from build123d import *

# Parameters (mm, degrees)
SKETCH1_R           = 1.720095417
SKETCH1_R_2         = 1.632335783
BOSS_EXTRUDE1_DEPTH = 2.54


with BuildPart() as part:
    # Sketch1 → Boss-Extrude1 (new body)
    with BuildSketch(Plane.XY):
        with BuildLine():
            Line((0.359622665, 84.647626996), (0.359622665, 112.547896558))
            ThreePointArc((0.359622665, 112.547896558), (1.569792033, 115.17822767), (4.285435965, 116.18243367))
            Line((4.285435965, 116.18243367), (699.960441306, 116.18243367))
            Line((699.960441306, 116.18243367), (699.960441306, 131.904163347))
            ThreePointArc((699.960441306, 131.904163347), (701.183091811, 134.700225562), (704.024750828, 135.812795653))
            Line((704.024750828, 135.812795653), (857.125984653, 135.812795653))
            Line((857.125984653, 135.812795653), (857.125984653, 124.543323228))
            Line((857.125984653, 124.543323228), (714.00720644, 124.543323228))
            Line((714.00720644, 124.543323228), (714.00720644, 104.995667719))
            Line((714.00720644, 104.995667719), (12.71320644, 104.995667719))
            Line((12.71320644, 104.995667719), (12.71320644, 91.663924817))
            Line((12.71320644, 91.663924817), (714.00720644, 91.663924817))
            Line((714.00720644, 91.663924817), (714.00720644, 72.51225313))
            Line((714.00720644, 72.51225313), (935.984655082, 72.51225313))
            Line((935.984655082, 72.51225313), (935.984655082, 124.543323228))
            Line((935.984655082, 124.543323228), (933.071984653, 124.543323228))
            Line((933.071984653, 124.543323228), (933.071984653, 135.812795653))
            Line((933.071984653, 135.812795653), (946.192785632, 135.812795653))
            ThreePointArc((946.192785632, 135.812795653), (948.657072186, 134.878542119), (949.738968911, 132.475411377))
            Line((949.738968911, 132.475411377), (949.738968911, 64.012598058))
            ThreePointArc((949.738968911, 64.012598058), (948.74540471, 61.39621374), (946.192785632, 60.24870663))
            Line((946.192785632, 60.24870663), (704.024750828, 60.24870663))
            ThreePointArc((704.024750828, 60.24870663), (701.213068629, 61.288906282), (699.960441306, 64.012598058))
            Line((699.960441306, 64.012598058), (699.960441306, 81.011908201))
            Line((699.960441306, 81.011908201), (4.285435965, 81.011908201))
            ThreePointArc((4.285435965, 81.011908201), (1.569547298, 82.016705042), (0.359622665, 84.647626996))
        make_face()
        with Locations((94.1622142, 88.091107164)):
            Circle(SKETCH1_R, mode=Mode.SUBTRACT)
        with Locations((94.1622142, 108.484732819)):
            Circle(SKETCH1_R, mode=Mode.SUBTRACT)
        with Locations((221.392126764, 108.484732819)):
            Circle(SKETCH1_R, mode=Mode.SUBTRACT)
        with Locations((221.392126764, 88.091107164)):
            Circle(SKETCH1_R, mode=Mode.SUBTRACT)
        with Locations((348.078760153, 108.484732819)):
            Circle(SKETCH1_R, mode=Mode.SUBTRACT)
        with Locations((348.078760153, 88.091107164)):
            Circle(SKETCH1_R_2, mode=Mode.SUBTRACT)
        with Locations((475.146430575, 108.484732819)):
            Circle(SKETCH1_R, mode=Mode.SUBTRACT)
        with Locations((475.146430575, 88.091107164)):
            Circle(SKETCH1_R, mode=Mode.SUBTRACT)
        with Locations((602.130384222, 88.091107164)):
            Circle(SKETCH1_R, mode=Mode.SUBTRACT)
        with Locations((602.130384222, 108.484732819)):
            Circle(SKETCH1_R, mode=Mode.SUBTRACT)
        with Locations((705.892847696, 116.18243367)):
            Circle(SKETCH1_R, mode=Mode.SUBTRACT)
        with Locations((705.892847696, 81.011908201)):
            Circle(SKETCH1_R, mode=Mode.SUBTRACT)
        with Locations((760.070975046, 130.611938178)):
            Circle(SKETCH1_R, mode=Mode.SUBTRACT)
        with Locations((760.070975046, 66.505299661)):
            Circle(SKETCH1_R, mode=Mode.SUBTRACT)
        with Locations((848.138968911, 130.611938178)):
            Circle(SKETCH1_R, mode=Mode.SUBTRACT)
        with Locations((848.138968911, 66.505299661)):
            Circle(SKETCH1_R, mode=Mode.SUBTRACT)
        with Locations((943.890172073, 116.18243367)):
            Circle(SKETCH1_R, mode=Mode.SUBTRACT)
        with Locations((943.890172073, 81.011908201)):
            Circle(SKETCH1_R, mode=Mode.SUBTRACT)
    extrude(amount=BOSS_EXTRUDE1_DEPTH)


solid = part.part
CAD build for the part. Positions are in the model's coordinates, mm. Round coordinates to 2 decimals unless told otherwise and drop trailing zeros. Write each loop counter-clockwise with the first axis right and the second up, starting at its lowest first coordinate (ties: lowest second). Pieces come first, ordered by that corner, then holes.
(1) Slice it at A-A, the plane x = 422.5. Write the cut outline in (y, z), and give its area (3 significant figures).
(2) Slice it at B-B, the plane x = 812. Write the cut outline in (y, z).
(3) Slice it at C-C, the plane z = 1.85. Count the separate pieces of the cut face and the enclosed holes in it, and give its area (3 significant figures).
(4) Probe line 1 along Y through (x, z) = (759.5, 0.9); line 2 along Y through (x, z) = (804, 1.55); line 3 along Y through (x, z) = (672.5, 0.75). List the from-to ranges inside material, lowest first.
From the geometry:
1. outline: (81.01, 0) - (91.66, 0) - (91.66, 2.54) - (81.01, 2.54) - close; (105, 0) - (116.18, 0) - (116.18, 2.54) - (105, 2.54) - close
1. area: 55.5 mm2
2. outline: (60.25, 0) - (72.51, 0) - (72.51, 2.54) - (60.25, 2.54) - close; (124.54, 0) - (135.81, 0) - (135.81, 2.54) - (124.54, 2.54) - close
3. separate pieces: 1
3. enclosed holes: 18
3. area: 21,500 mm2
4. line 1: y = 60.25 to 64.88, 68.13 to 72.51, 124.54 to 128.99, 132.23 to 135.81
4. line 2: y = 60.25 to 72.51, 124.54 to 135.81
4. line 3: y = 81.01 to 91.66, 105 to 116.18
